Model file for the job. Use its own axes, mm. A direction names the side the tool comes from. Round coordinates to 2 decimals unless told otherwise and drop trailing zeros. Order: outer loops, then holes, each group sorted by start corner. A loop starts at its lowest first (then second) coordinate and runs counter-clockwise, first axis right, second up. Notation, with made-up numbers: (36, 86.25) -> (88, 86.25) arc R18 cw to (88, 92.25) -> close; hole circle Ø5 at (60.25, -20). An arc over 180 degrees is marked (long way). Use CSV: the item, a comma, the result in double quotes.
Autodesk Inventor part; units mm, degrees
ref_plane "Piano di lavoro1" through (-90, 0, -15) normal (-1, 0, 0) x (0, -1, 0)
ref_plane "Piano di lavoro3" through (0, 0, -30) normal (0, 0.4988877, -0.8666667) x (-1, 0, 0)
ref_plane "YZ Plane" through (0, 0, 0) normal (1, 0, 0) x (0, 1, 0)
sketch "Schizzo1" plane through (0, 0, 0) normal (0, 1, 0) x (-1, 0, 0)
  line L0 (0, 0) -> (0, -30)
  line L1 (0, -15) -> (90, -15)
  line L2 (100, 0) -> (100, -30)
  line L3 (0, -30) -> (100, -30)
  line L4 (100, 0) -> (0, 0)
  line L5 (100, -41.4573) -> (75, -41.4573)
  line L6 (75, -17) -> (85, -17)
  line L7 (75, -17) -> (75, -22)
  line L8 (85, -17) -> (85, -29.5)
  line L9 (75, -22) -> (80, -22)
  line L10 (80, -22) -> (80, -24.5)
  line L11 (80, -24.5) -> (5, -24.5)
  line L12 (85, -29.5) -> (5, -29.5)
  line L13 (5, -24.5) -> (5, -29.5)
  dimension "d0" = 30
  dimension "d1" = 90
  dimension "d5" = 25
  dimension "d6" = 17
  dimension "d7" = 10
  dimension "d8" = 5
  dimension "d9" = 12.5
  dimension "d10" = 5
  dimension "d11" = 2.5
  dimension "d13" = 80
  dimension "d16" = 75
  dimension "d76" = 100
sketch "Schizzo2" plane through (0, 0, 0) normal (1, 0, 0) x (0, 1, 0)
  circle A0 centre (0, -15) radius 13
  circle A1 centre (0, -15) radius 12
  line L0 (5, -4.0913) -> (-5, -4.0913)
  line L1 (-5, -4.0913) -> (-5, -25.9087)
  line L2 (-5, -25.9087) -> (5, -25.9087)
  line L3 (5, -25.9087) -> (5, -4.0913)
  point P0 (0, 0)
  dimension "d2" = 15
  dimension "d3" = 26
  dimension "d53" = 24
  dimension "d58" = 10
  dimension "d59" = 21.8174
ref_plane "Piano di lavoro1" through (-90, 0, -15) normal (-1, 0, 0) x (0, -1, 0)
sketch "Schizzo3" plane through (-90, 0, -15) normal (-1, 0, 0) x (0, -1, 0)
  circle A0 centre (0, 0) radius 13
  point P0 (0, 15)
  dimension "d4" = 26
loft "Loft1" add profiles "Schizzo3", "Schizzo2" contours all / A0 | A1 L3 | L0 A1 | L3 L2 L1 L0 | A1 L2 | L1 A1
shell "Svuotamento1" thickness 3 removed faces 2 at (0, 3.4665, -13.963) at (-90, -3.4665, -13.963)
ref_plane "Piano di lavoro3" through (0, 0, -30) normal (0, 0.4988877, -0.8666667) x (-1, 0, 0)
sketch "Schizzo11" plane through (0, 0, -30) normal (0, 0.4988877, -0.8666667) x (-1, 0, 0)
  point P0 (0, 14.9666)
extrude "Estrusione5" add sketch "Schizzo2" against normal blind 10 contours A1 L3 | L0 A1 | L3 L2 L1 L0 | A1 L2 | L1 A1
extrude "Estrusione6" add sketch "Schizzo2" along normal blind 31.4 contours L3 L2 L1 L0
fillet "Raccordo1" radius 10 1 edges at (31.4, 0, -25.9087)
fillet "Raccordo2" radius 10 1 edges at (31.4, 0, -4.0913)
sketch "Schizzo12" plane through (0, -5, -25.9087) normal (0, -1, 0) x (1, 0, 0)
  line L0 (0, 0) -> (21.4, 0)
  line L1 (6.4, 21.8172) -> (21.4, 21.8172)
  line L2 (31.4, 11.8174) -> (31.4, 10)
  circle A0 centre (18.9, 10.9087) radius 5
  line L3 (0, 25.9087) -> (0, -2.0913)
  point P0 (13.9, 21.8172)
  point P1 (31.4, 10.9087)
  point P2 (10.7, 0)
  point P3 (31.4, 10.9087)
  point P4 (0, -2.0913)
  dimension "d64" = 21.8172
  dimension "d70" = 10
  dimension "d71" = 12.5
  dimension "d72" = 10.9085
  dimension "d75" = 18.9
extrude "Estrusione7" cut sketch "Schizzo12" against normal blind 25
fillet "Raccordo3" radius 5 1 edges at (0, 13, -15)
sketch "Schizzo13" plane through (0, 0, 0) normal (0, 0, 1) x (1, 0, 0)
  line L0 (-33, 8.7721) -> (-83, 8.7721)
  line L1 (-90, 10) -> (-10, 10)
  line L2 (-33, 8.7721) -> (-33, 5)
  line L3 (-5, -13) -> (-5, 13)
  line L4 (-83, 8.7721) -> (-83, -10)
  line L5 (-83, -10) -> (-69.4203, -10)
  line L6 (-90, -10) -> (-10, -10)
  line L7 (-69.4203, -10) -> (-69.4203, 2.7972)
  line L8 (-69.4203, 2.7972) -> (-74.4203, 2.7972)
  line L9 (-74.4203, 2.7972) -> (-74.4203, -5)
  line L10 (-74.4203, -5) -> (-78, -5)
  line L11 (-78, -5) -> (-78, 5)
  line L12 (-33, 5) -> (-78, 5)
  point P0 (0, 0)
  point P1 (-33, 6.8861)
  dimension "d21" = 3
  dimension "d79" = 28
  dimension "d80" = 50
  dimension "d83" = 5
  dimension "d84" = 5
  dimension "d85" = 7.7972
  dimension "d86" = 5
  dimension "d87" = 5
extrude "Estrusione8" cut sketch "Schizzo13" against normal blind 10
properties part number "asteoscila1_(306)"
Q1. Cut at A-A (x = 18.9). Give the cut face in (y, z).
From the geometry:
outline,"(-5, -25.91) -> (5, -25.91) -> (5, -20) -> (-5, -20) -> close; (-5, -10) -> (5, -10) -> (5, -4.09) -> (-5, -4.09) -> close"
Q2. Which spindle directions (+Z, -Z, +X, -X, +Y, -Y) get a long thin tool onto all of the face, cutting with end or side? Do faces 1 (the flat face through (-55, 5, -5)), 2 (the cylindrical face through (-49.44, -5.38, -23.43)), 3 (the flat face through (-72, 2.797, -4)), 4 (the flat face through (0, 6, -15)), 5 (the flat face through (0, -6, -15)). Say none if no direction does.
From the geometry:
face 1,"+Z"
face 2,"-X"
face 3,"+Z, -Y"
face 4,"+Z, -Z, +X, +Y"
face 5,"+Z, -Z, +X, -Y"
Q3. Cut at D-D (x = -19). Give the cut face in (y, z).
From the geometry:
outline,"circle Ø26 at (0, -15); hole circle Ø20 at (0, -15)"
Q4. Cut at B-B (y = 0). Give the cut face in (x, z).
From the geometry:
outline,"(-90, -28) -> (-5, -28) arc R5 ccw to (-0.93, -25.91) -> (21.4, -25.91) arc R10 ccw to (31.4, -15.91) -> (31.4, -14.09) arc R10 ccw to (21.4, -4.09) -> (-0.93, -4.09) arc R5 ccw to (-5, -2) -> (-69.42, -2) -> (-69.42, -5) -> (-10, -5) -> (-10, -25) -> (-90, -25) -> close; (-90, -5) -> (-83, -5) -> (-83, -2) -> (-90, -2) -> close; (-78, -5) -> (-74.42, -5) -> (-74.42, -2) -> (-78, -2) -> close; hole circle Ø10 at (18.9, -15)"
Q5. Cut at C-C (x = -50). Give the cut face in (y, z), plus the area to 3 significant figures.
From the geometry:
outline,"(5, -6.34) -> (5, -3) arc R13 ccw (long way) to (8.77, -5.41) -> (8.77, -10) -> (8.66, -10) arc R10 cw (long way) to start"
area,"202 mm²"
Q6. Mould opens along Y. For faces 6 (the flat face through (-76, -5, -5)), 7 (the flat face through (-33, 7, -6)), 8 (the cylindrical face through (21.207, -0.07, -19.436)) say: +Y half, -Y half, draft (parallel to the pull), parting line (faces both ways), or undercut.
From the geometry:
face 6,"-Y half"
face 7,"undercut"
face 8,"draft"
Q7. Pin check, flat tips, straight feed: pin 1 (5 mm diameter, centred on y = 9, z = -20.5, fed in from +X); pin 2 (0.7 mm diameter, centred on x = -77.5, y = -9.5, fed in from +Z); pin 3 (1.7 mm diameter, centred on x = -75.5, z = -5.5, fed in from -Y); pin 4 (5 mm diameter, centred on x = -34, y = 0.5, fed in from +Z). Stop position of each tip, or through.
From the geometry:
pin 1,"stops at x = 0"
pin 2,"stops at z = -10"
pin 3,"stops at y = -5"
pin 4,"stops at z = -2"
Q8. Probe line 1 along Y through (x, z) = (-68, -15); line 2 along Z through (x, y) = (18.9, -0.5); line 3 along Z through (x, y) = (-64, 0). List the from-to ranges inside material, lowest first.
From the geometry:
line 1,"y = -13 to -10, 10 to 13"
line 2,"z = -25.91 to -20, -10 to -4.09"
line 3,"z = -28 to -25, -5 to -2"
